Can you work these out from the drawing? Everything is in mm from the part's minimum corner. Coordinates: 2 decimals unless noted, no trailing zeros. Loops run counter-clockwise (first coordinate to the right, second up) from the corner with the lowest first, then second, coordinate; pieces in that order, holes last. Notation, with made-up numbers: (35, 50.5) - (64, 50.5) arc R23 cw to (64, 83.5) - close; hole circle Ø5 at (78.25, 41.25). An arc over 180 degrees is marked (long way). Put each result on its own line as item: value. Start each with the question number.
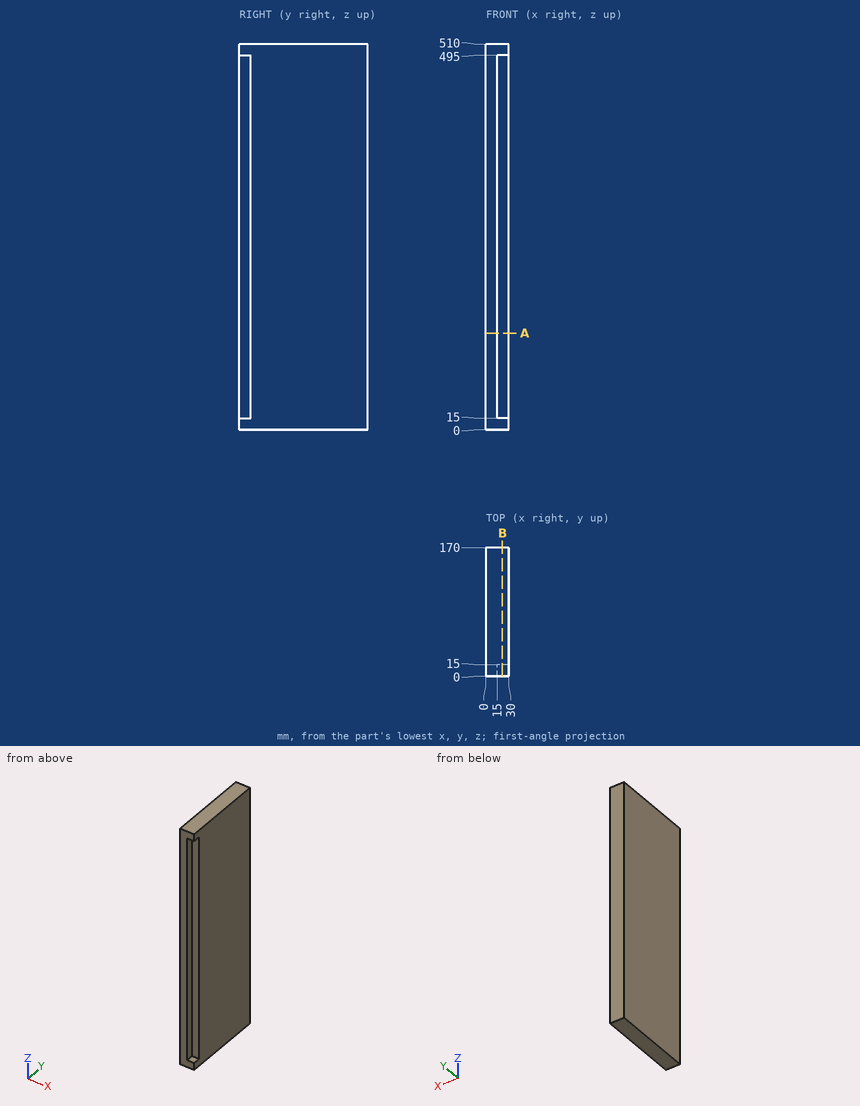
Q1. I want a section at B-B on x = 21.75. List the corners of the cut face in (y, z) for me, and give its area (3 significant figures).
Q2. Will these pins go through, and if not, where does the flat tip stop? pin 1 (6 mm diameter, centred on x = 21, z = 195, fed in from -Y); pin 2 (4.5 mm diameter, centred on x = 22, y = 4, fed in from -Z); pin 3 (4.5 mm diameter, centred on y = 6, z = 188, fed in from +X).
Q3. I want a section at A-A on z = 127.5. List the corners of the cut face in (x, y) for me.
Q4. Please list where these lines run through material, in increasing order: line 1 along Y through (x, z) = (23, 68); line 2 along X through (y, z) = (9.5, 247). Write a range as [from, to].
Calculated:
1. outline: (0, 0) - (170, 0) - (170, 510) - (0, 510) - (0, 495) - (15, 495) - (15, 15) - (0, 15) - close
1. area: 79,500 mm2
2. pin 1: y = 15
2. pin 2: z = 0
2. pin 3: x = 15
3. outline: (0, 0) - (15, 0) - (15, 15) - (30, 15) - (30, 170) - (0, 170) - close
4. line 1: [15, 170]
4. line 2: [0, 15]
